Part print with two shaded views. Sizes in mm from the minimum x, y, z corner. A direction names the side the tool comes from. Coordinates: 2 decimals unless noted, no trailing zeros. Write each loop counter-clockwise with the first axis right and the second up, starting at its lowest first coordinate (ties: lowest second). Pieces come first, ordered by that corner, then holes. Notation, with made-up numbers: (-38.5, 74) - (11.5, 74) arc R11 ccw to (11.5, 78) - close; hole circle Ø11 at (15.5, 23). An arc over 180 degrees is marked (long way). Answer in a Markdown table with one row per item. Add a question column.
Q1. Pin check, flat tips, straight feed: pin 1 (2 mm diameter, centred on y = 8, z = 80.5, fed in from -X); pin 2 (4 mm diameter, centred on y = 2.5, z = 10.5, fed in from -X); pin 3 (8 mm diameter, centred on y = 9.5, z = 39.5, fed in from +X). Stop position of each tip, or through.
Q2. 3-axis set-ups, long thin cutter, end or side, ignore diameter. For the marked faces 1, 2 and 3: which of +Z, -Z, +X, -X, +Y, -Y reach the whole face in a straight line?
Q3. Band-saw the part on A-A (y = 10.5). List the corners of the cut face in (x, z), and give its area (3 significant figures).
Q4. Band-saw the part on C-C (x = 10.5). List the corners of the cut face in (y, z), and give its area (3 significant figures).
Q5. Band-saw the part on D-D (y = 15.25). List the corners of the cut face in (x, z).
Q6. Band-saw the part on B-B (z = 16.5). List the corners of the cut face in (x, y).
Q7. Drill centre lines: line 1 along X through (y, z) = (7, 63); line 2 along X through (y, z) = (6.25, 77); line 3 along Y through (x, z) = (5.5, 27). Where is each one in solid material? Low to high. Write a range as from..to.
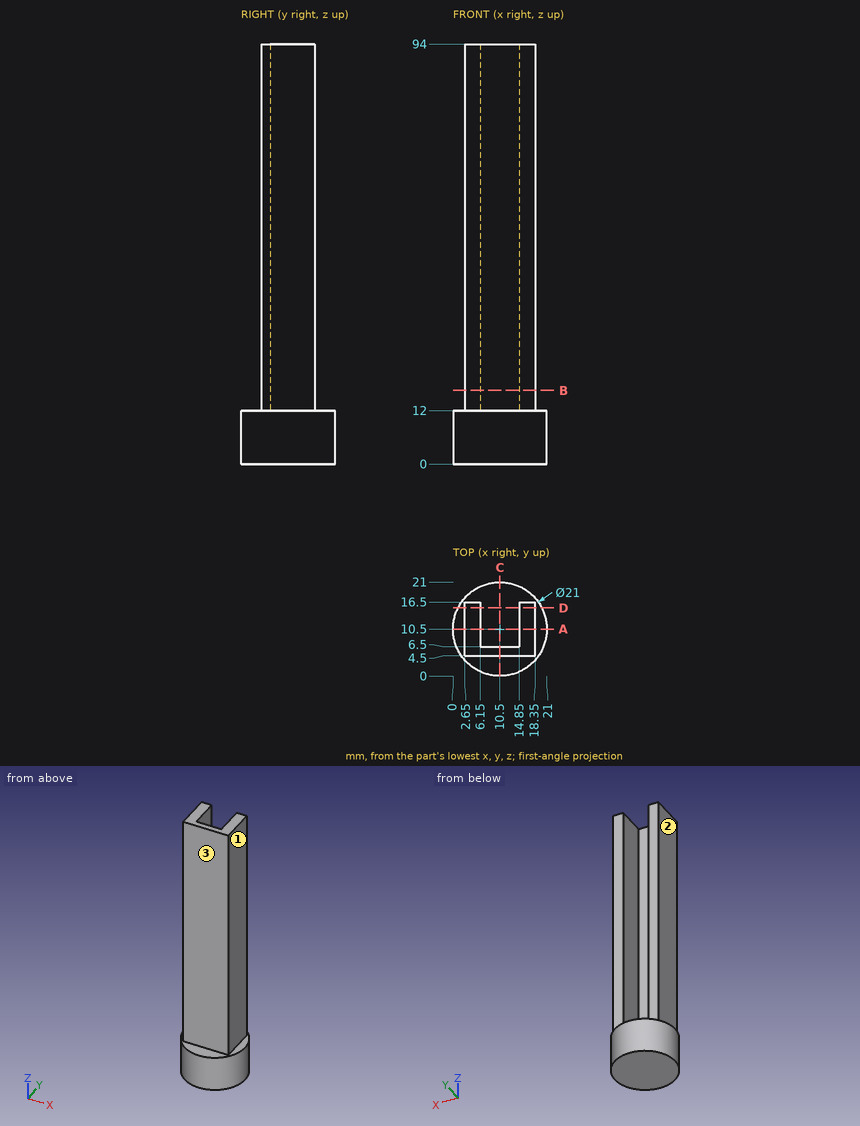
Checked values:
| question | item | result |
|---|---|---|
| 1 | pin 1 | stops at x = 2.65 |
| 1 | pin 2 | stops at x = 1.88 |
| 1 | pin 3 | stops at x = 18.35 |
| 2 | face 1 | +Z, +X, +Y, -Y |
| 2 | face 2 | +Z, -X, +Y, -Y |
| 2 | face 3 | +Z, +X, -X, -Y |
| 3 | outline | (0, 0) - (21, 0) - (21, 12) - (18.35, 12) - (18.35, 94) - (14.85, 94) - (14.85, 12) - (6.15, 12) - (6.15, 94) - (2.65, 94) - (2.65, 12) - (0, 12) - close |
| 3 | area | 826 mm² |
| 4 | outline | (0, 0) - (21, 0) - (21, 12) - (6.5, 12) - (6.5, 94) - (4.5, 94) - (4.5, 12) - (0, 12) - close |
| 4 | area | 416 mm² |
| 5 | outline | (1.14, 0) - (19.86, 0) - (19.86, 12) - (18.35, 12) - (18.35, 94) - (14.85, 94) - (14.85, 12) - (6.15, 12) - (6.15, 94) - (2.65, 94) - (2.65, 12) - (1.14, 12) - close |
| 6 | outline | (2.65, 4.5) - (18.35, 4.5) - (18.35, 16.5) - (14.85, 16.5) - (14.85, 6.5) - (6.15, 6.5) - (6.15, 16.5) - (2.65, 16.5) - close |
| 7 | line 1 | x = 2.65..6.15, 14.85..18.35 |
| 7 | line 2 | x = 2.65..18.35 |
| 7 | line 3 | y = 4.5..16.5 |
